CAD build for the part. Positions are in the model's coordinates, mm. Face numbers are marked on the shaded views. A direction names the side the tool comes from. Give positions to 0.01 mm unless a question says otherwise; leave off trailing zeros. Order: outer loops, then holes, each group sorted by start corner. A loop starts at its lowest first (then second) coordinate and runs counter-clockwise, first axis right, second up.
Autodesk Inventor part; units mm, degrees
ref_plane "YZ Plane" through (0, 0, 0) normal (1, 0, 0) x (0, 1, 0)
ref_plane "XZ Plane" through (0, 0, 0) normal (0, 1, 0) x (-1, 0, 0)
ref_plane "XY Plane" through (0, 0, 0) normal (0, 0, 1) x (1, 0, 0)
sketch "Sketch1" plane through (0, 0, 0) normal (0, 0, 1) x (1, 0, 0)
  line L0 (0, 0) -> (33.5, 0)
  line L1 (33.5, 0) -> (33.5, -115)
  line L2 (33.5, -115) -> (0, -115)
  line L3 (0, -115) -> (0, 0)
  dimension "d0" = 115
  dimension "d1" = 33.5
extrude "Extrusion1" add sketch "Sketch1" along normal blind 43
fillet "Fillet1" radius 2 12 edges at (33.5, -57.5, 0) (33.5, 0, 21.5) (33.5, -57.5, 43) (33.5, -115, 21.5) (16.75, -115, 0) (16.75, -115, 43) (0, -115, 21.5) (0, -57.5, 0) (0, -57.5, 43) (0, 0, 21.5) (16.75, 0, 0) (16.75, 0, 43)
sketch "Sketch2" plane through (2, -115, 41) normal (0, -1, 0) x (1, 0, 0)
  line L0 (0, -39) -> (0, 0)
  line L1 (0, -26.5048) -> (8.8714, -26.5048)
  line L2 (8.8714, -26.5048) -> (8.8714, -12.339)
  line L3 (8.8714, -12.339) -> (0, -12.339)
  line L4 (0, -12.339) -> (0, -26.5048)
  line L5 (25.0138, -23.8693) -> (29.2965, -23.8693)
  line L6 (29.2965, -23.8693) -> (29.2965, -12.339)
  line L7 (29.2965, -12.339) -> (25.0138, -12.339)
  line L8 (25.0138, -12.339) -> (25.0138, -23.8693)
  point P0 (-2, -41)
  point P1 (0, -12.339)
extrude "Extrusion2" add sketch "Sketch2" along normal blind 10
properties part number "battery2500"
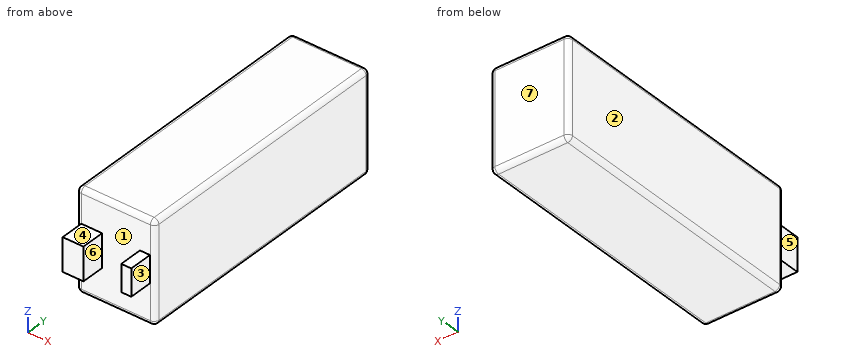
Item 1: Slice it at B-B (z = 35). Give the cut face in (x, y), and give its area (3 significant figures).
Item 2: Two-plate mould, pull along X, no slides. Class the marked faces 1, 2 and 3: released by +X, released by -X, zero draft, split by the parting line, or undercut.
Item 3: Wall check: L1, parallel to X at y = -118, z = 19; L2, parallel to Y at x = 25, z = 29.5. Give the ranges that are in metal, low to high.
Item 4: Slice it at D-D (z = 25.5). Give the cut face in (x, y), and give its area (3 significant figures).
Item 5: Slice it at C-C (x = 4). Give the cut face in (y, z), and give its area (3 significant figures).
Item 6: Slice it at A-A (x = 30). Give the cut face in (y, z).
Item 7: Drop flat-ended pins along their axis: pin 1 Ø2 at (x, z) = (23.5, 21) entering from -Y; pin 2 Ø11 at (y, z) = (-120, 23) entering from +X; pin 3 Ø3.5 at (x, y) = (29, -117.5) entering from -Z. Give the stop position or say it passes through.
Item 8: Tool access for the marked faces 4, 5, 6 and 7: list every direction of +Z, -Z, +X, -X, +Y, -Y with a clear straight run to the whole face (end or side of a thin tool).
A:
1. outline: (0, -113) arc R2 ccw to (2, -115) - (31.5, -115) arc R2 ccw to (33.5, -113) - (33.5, -2) arc R2 ccw to (31.5, 0) - (2, 0) arc R2 ccw to (0, -2) - close
1. area: 3,850 mm2
2. face 1: undercut
2. face 2: released by -X
2. face 3: released by +X
3. L1: x = 2 to 10.87, 27.01 to 31.3
3. L2: y = -115 to 0
4. outline: (0, -113) arc R2 ccw to (2, -115) - (2, -125) - (10.87, -125) - (10.87, -115) - (27.01, -115) - (27.01, -125) - (31.3, -125) - (31.3, -115) - (31.5, -115) arc R2 ccw to (33.5, -113) - (33.5, -2) arc R2 ccw to (31.5, 0) - (2, 0) arc R2 ccw to (0, -2) - close
4. area: 3,980 mm2
5. outline: (-125, 14.5) - (-115, 14.5) - (-115, 2) arc R2 ccw to (-113, 0) - (-2, 0) arc R2 ccw to (0, 2) - (0, 41) arc R2 ccw to (-2, 43) - (-113, 43) arc R2 ccw to (-115, 41) - (-115, 28.66) - (-125, 28.66) - close
5. area: 5,080 mm2
6. outline: (-125, 17.13) - (-115, 17.13) - (-115, 2) arc R2 ccw to (-113, 0) - (-2, 0) arc R2 ccw to (0, 2) - (0, 41) arc R2 ccw to (-2, 43) - (-113, 43) arc R2 ccw to (-115, 41) - (-115, 28.66) - (-125, 28.66) - close
7. pin 1: stops at y = -115
7. pin 2: stops at x = 32.82
7. pin 3: stops at z = 17.13
8. face 4: +Z, +X, -X, -Y
8. face 5: +Z, -Z, -X, -Y
8. face 6: +Z, -Z, -Y
8. face 7: +Z, -Z, +X, -X, +Y
